Part model, mm, in its own coordinate system. Face numbers are marked on the shaded views. A direction names the side the tool comes from. Coordinates: 2 decimals unless noted, no trailing zeros. Order: outer loops, then holes, each group sorted by start corner. A loop starts at its lowest first (then second) coordinate and runs counter-clockwise, first axis right, second up. Notation, with made-up numbers: (56, 88) - (100, 88) arc R23 cw to (100, 108) - close; hole circle Ø11 at (88.25, 89.25). An arc over 180 degrees is marked (long way). Use a Markdown table: item, result. Add a question column.
1) Saw through at B-B on x = -27.5. List the corners of the cut face in (y, z), then the cut area to 3 significant figures.
2) Saw through at C-C on y = 2. List the corners of the cut face in (x, z).
3) Drop flat-ended pins along their axis: P1, Ø2.5, axis at y = 15.5, z = 5, coming from the +X side; P2, Ø2, axis at x = 0, z = 10, coming from the -Y side; P3, Ø6.5, axis at x = 25.89, z = 6, coming from the -Y side. Give the stop position or say it passes through.
4) Tool access for the marked faces 1, 2 and 3: list every direction of +Z, -Z, +X, -X, +Y, -Y with a clear straight run to the whole face (end or side of a thin tool).
5) Saw through at A-A on z = 6. Count the separate pieces of the cut face and the enclosed holes in it, then the cut area to 3 significant figures.
6) Wall check: L1, parallel to X at y = -3, z = 3.5; L2, parallel to Y at x = -2.5, z = 0.5; L3, parallel to Y at x = -24.5, z = 7.75. Give the ranges that are in metal, low to high. Write a range as [from, to].
7) Two-plate mould, pull along Y, no slides. Class the marked faces 4, 5, 6 and 7: +Y half, -Y half, draft (parallel to the pull), parting line (faces both ways), or undercut.
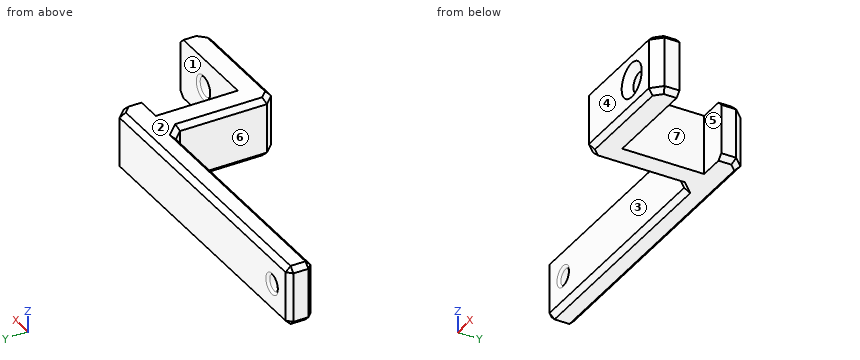
```python
from build123d import *

# Parameters (mm, degrees)
RESSALTO_EXTRUS_O1_DEPTH = 12
ESBO_O3_R                = 2
CORTE_EXTRUS_O1_DEPTH    = 15
CHANFRO1_SIZE            = 1.5
FILETE1_R                = 0.5
CHANFRO5_SIZE            = 2
CHANFRO8_SIZE            = 1
ESBO_O4_R                = 1.65
CORTE_EXTRUS_O2_DEPTH    = 10
FILETE2_R                = 0.5


with BuildPart() as part:
    # Esboço1 → Ressalto-extrusão1 (new body)
    with BuildSketch(Plane.XY):
        Polygon((19.886382163, 14.25), (13.886382163, 14.25), (13.886382163, -2.25), (33.886382163, -2.25), (33.886382163, -7.25), (8.886382163, -7.25), (8.886382163, 14.25), (-41.113617837, 14.25), (-41.113617837, 19.25), (19.886382163, 19.25), align=None)
    extrude(amount=RESSALTO_EXTRUS_O1_DEPTH)

    # Esboço3 → Corte-extrusão1 (cut)
    with BuildSketch(Plane.XZ.offset(7.25)):
        with Locations(Location((25.886382163, 6, 0), (0, 0, 270))):
            Circle(ESBO_O3_R)
    extrude(amount=-CORTE_EXTRUS_O1_DEPTH, mode=Mode.SUBTRACT)

    # Chanfro1
    chanfro1_edges = [part.edges().sort_by_distance(p)[0] for p in [
        (25.886382163, -7.25, 8),
    ]]
    chamfer(chanfro1_edges, length=CHANFRO1_SIZE)

    # Filete1
    filete1_edges = [part.edges().sort_by_distance(p)[0] for p in [
        (25.886382163, -2.25, 8),
    ]]
    fillet(filete1_edges, radius=FILETE1_R)

    # Chanfro5
    chanfro5_edges = [part.edges().sort_by_distance(p)[0] for p in [
        (33.886382163, -7.25, 6),
        (8.886382163, -7.25, 6),
        (8.886382163, 14.25, 6),
        (19.886382163, 19.25, 6),
    ]]
    chamfer(chanfro5_edges, length=CHANFRO5_SIZE)

    # Chanfro8
    chanfro8_edges = [part.edges().sort_by_distance(p)[0] for p in [
        (-41.113617837, 19.25, 6),
        (-41.113617837, 16.75, 12),
        (-41.113617837, 14.25, 6),
        (-41.113617837, 16.75, 0),
        (19.886382163, 15.75, 0),
        (-11.613617837, 19.25, 0),
        (33.886382163, -3.75, 0),
        (32.886382163, -6.25, 0),
        (21.386382163, -7.25, 0),
        (9.886382163, -6.25, 0),
        (8.886382163, 3.5, 0),
        (7.886382163, 13.25, 0),
        (-17.113617837, 14.25, 0),
        (33.886382163, -3.75, 12),
        (32.886382163, -6.25, 12),
        (21.386382163, -7.25, 12),
        (9.886382163, -6.25, 12),
        (8.886382163, 3.5, 12),
        (7.886382163, 13.25, 12),
        (-17.113617837, 14.25, 12),
        (19.886382163, 15.75, 12),
        (-11.613617837, 19.25, 12),
        (18.886382163, 18.25, 0),
        (18.886382163, 18.25, 12),
    ]]
    chamfer(chanfro8_edges, length=CHANFRO8_SIZE)

    # Esboço4 → Corte-extrusão2 (cut)
    with BuildSketch(Plane(origin=(0, 19.25, 0), x_dir=(1, 0, 0), z_dir=(0, 1, 0))):
        with Locations(Location((-35.363617837, -6, 0), (0, 0, 270))):
            Circle(ESBO_O4_R)
    extrude(amount=-CORTE_EXTRUS_O2_DEPTH, mode=Mode.SUBTRACT)

    # Filete2
    filete2_edges = [part.edges().sort_by_distance(p)[0] for p in [
        (-35.363617837, 14.25, 4.35),
        (-35.363617837, 19.25, 4.35),
    ]]
    fillet(filete2_edges, radius=FILETE2_R)


solid = part.part
```
Results are:
| question | item | result |
|---|---|---|
| 1 | outline | (14.25, 1) - (15.25, 0) - (18.25, 0) - (19.25, 1) - (19.25, 11) - (18.25, 12) - (15.25, 12) - (14.25, 11) - close |
| 1 | area | 58.0 mm2 |
| 2 | outline | (8.89, 1) - (9.89, 0) - (13.89, 0) - (13.89, 12) - (9.89, 12) - (8.89, 11) - close |
| 3 | P1 | x = 19.89 |
| 3 | P2 | y = 14.25 |
| 3 | P3 | y = -7 |
| 4 | face 1 | +Z, -Z, +X |
| 4 | face 2 | +Z, +X, -X, +Y, -Y |
| 4 | face 3 | +Z, -Z, -X, -Y |
| 5 | separate pieces | 3 |
| 5 | enclosed holes | 0 |
| 5 | area | 468 mm2 |
| 6 | L1 | [8.89, 33.89] |
| 6 | L2 | [14.75, 18.75] |
| 6 | L3 | [14.25, 19.25] |
| 7 | face 4 | -Y half |
| 7 | face 5 | undercut |
| 7 | face 6 | draft |
| 7 | face 7 | undercut |
